For this review, use the dimensioned drawing (mm, ordinates from the lowest corner) and the shaded views. Round coordinates to 2 decimals unless told otherwise and drop trailing zeros. Write each loop counter-clockwise with the first axis right and the second up, starting at its lowest first coordinate (ties: lowest second). Pieces come first, ordered by that corner, then holes. Notation, with made-up numbers: (-16, 34.25) -> (-12, 34.25) arc R15 cw to (-12, 49.25) -> close; hole circle Ø3 at (57.25, 54.25). An arc over 180 degrees is marked (long way). Write each question's results on one line, items separated by ' | '. Start each with the question number.
Item 1: Add section C-C (z = 7.75). State the section outline as (x, y) points.
Item 2: Add section B-B (x = 55). State the section outline as (y, z) points, plus the area to 3 significant figures.
Item 3: To check wall thickness, follow line 1 along Z through (x, y) = (60.5, 10); line 2 along Y through (x, z) = (46, 8.25); line 3 along X through (y, z) = (8, 15). State the ranges of each line that lie inside material, in increasing order.
Item 4: Clearance check with flat-ended pins moving along their axes: pin 1 (1.2 mm diameter, centred on y = 7, z = 15.5, fed in from +X); pin 2 (5.5 mm diameter, centred on x = 57.5, y = 9, fed in from +Z); pin 3 (4.5 mm diameter, centred on y = 6.5, z = 4, fed in from +X). State where each tip first meets the part, or that it passes through.
Item 5: Add section A-A (y = 6.5). State the section outline as (x, z) points, plus the area to 3 significant figures.
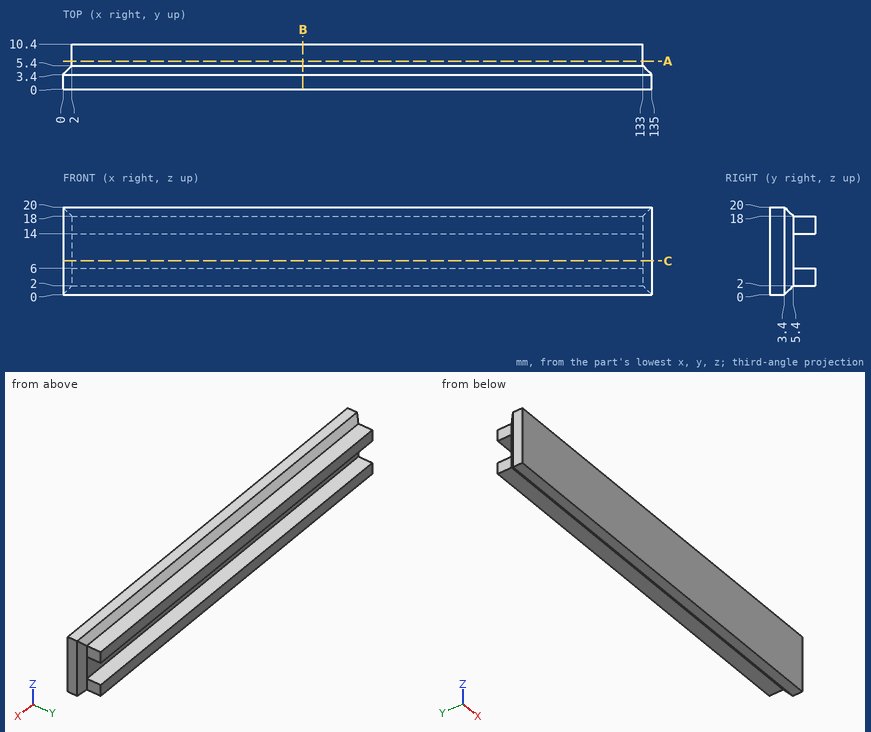
Responses:
1) outline: (0, 0) -> (135, 0) -> (135, 3.4) -> (133, 5.4) -> (2, 5.4) -> (0, 3.4) -> close
2) outline: (0, 0) -> (3.4, 0) -> (5.4, 2) -> (10.4, 2) -> (10.4, 6) -> (5.4, 6) -> (5.4, 14) -> (10.4, 14) -> (10.4, 18) -> (5.4, 18) -> (3.4, 20) -> (0, 20) -> close | area: 144 mm^2
3) line 1: z = 2 to 6, 14 to 18 | line 2: y = 0 to 5.4 | line 3: x = 2 to 133
4) pin 1: stops at x = 133 | pin 2: stops at z = 18 | pin 3: stops at x = 134.15
5) outline: (2, 2) -> (133, 2) -> (133, 6) -> (2, 6) -> close; (2, 14) -> (133, 14) -> (133, 18) -> (2, 18) -> close | area: 1,050 mm^2
